Design review of the part shown in the three views and the two pictorial views. Dimensions are in mm from the part's minimum x, y and z. A direction names the side the tool comes from. Round coordinates to 2 decimals unless told otherwise and drop trailing zeros. Loops run counter-clockwise (first coordinate to the right, second up) from the corner with the lowest first, then second, coordinate; pieces in that order, holes last. Notation, with made-up numbers: M -6.75,54.5 L 52.25,54.5 A18 cw 52.25,68.5 Z; hole C 12,-22.5 d8. An arc over 180 degrees is marked long. One line per question, with ' | ' between items. Start each with the question number.
1) For the marked faces 5, 6, 7 and 8, list the 3-axis set-ups (+Z, -Z, +X, -X, +Y, -Y) from which the entire face can be reached by the end or side of a thin tool; tool diameter is ignored.
2) Mouldability with a two-part tool opening along X and no side actions: class the marked faces 1, 2, 3 and 4 as pulls with the +X half, pulls with the -X half, needs draft (parallel to the pull), parting line crosses it, or undercut.
3) We need section C-C (x = 29). Give the boundary of the cut face in (y, z).
4) For probe 1 along X at (y, z) = (1.25, 7.5); probe 2 along X at (y, z) = (4, 1); probe 3 along X at (y, z) = (3, 2.5), list the stretches that pass through material, from the lowest coordinate up. Write a range as from..to.
5) For pin 1 Ø4.5 at (x, z) = (28, 3) entering from +Y (1 decimal); pin 2 Ø2.5 at (x, z) = (5, 14) entering from +Y, all flat-tipped, find the tip position at first contact; note any pin that passes through.
6) We need section A-A (x = 7). Give the boundary of the cut face in (y, z).
7) We need section D-D (z = 1). Give the boundary of the cut face in (x, y).
8) We need section B-B (z = 11.5). Give the boundary of the cut face in (x, y), and give its area (3 significant figures).
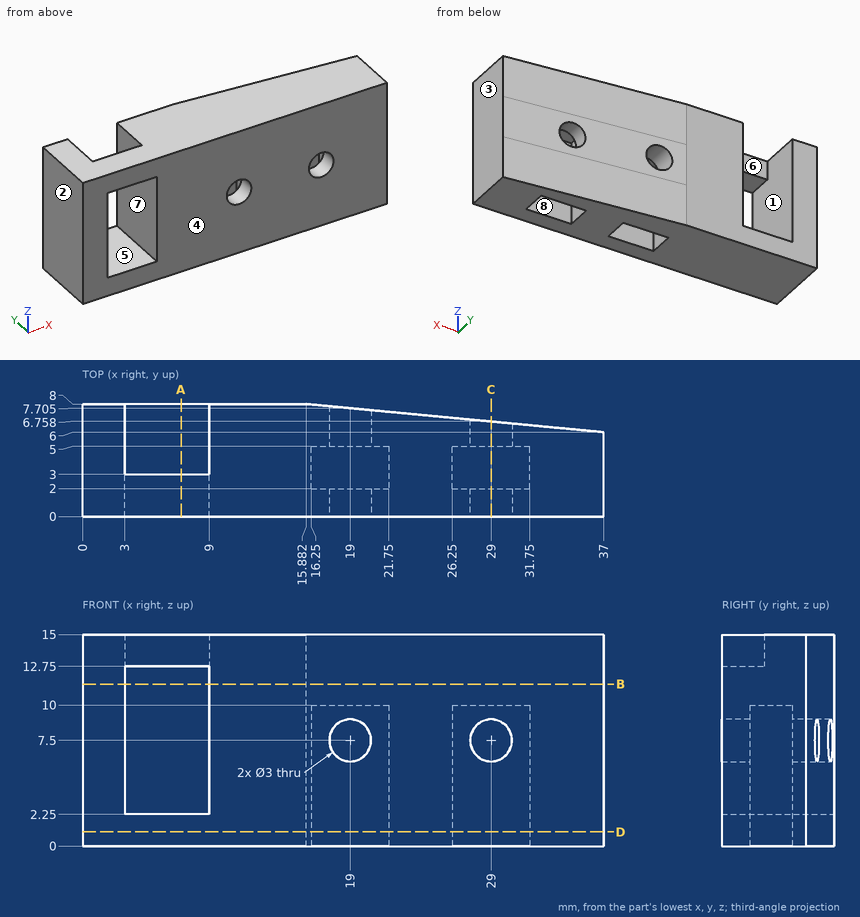
Answers below:
1) face 5: +Y, -Y | face 6: +Z, +Y | face 7: +Y | face 8: -Z
2) face 1: undercut | face 2: pulls with the -X half | face 3: pulls with the +X half | face 4: needs draft
3) outline: M 0,0 L 2,0 L 2,6 L 0,6 Z; M 0,9 L 2,9 L 2,10 L 5,10 L 5,9 L 6.76,9 L 6.76,15 L 0,15 Z; M 5,0 L 6.76,0 L 6.76,6 L 5,6 Z
4) probe 1: 0..3, 9..17.5, 20.5..27.5, 30.5..37 | probe 2: 0..16.25, 21.75..26.25, 31.75..37 | probe 3: 0..3, 9..16.25, 21.75..26.25, 31.75..37
5) pin 1: y = 7.1 | pin 2: y = 3
6) outline: M 0,0 L 8,0 L 8,2.25 L 0,2.25 Z; M 0,12.75 L 3,12.75 L 3,15 L 0,15 Z
7) outline: M 0,0 L 37,0 L 37,6 L 15.88,8 L 0,8 Z; hole M 16.25,2 L 21.75,2 L 21.75,5 L 16.25,5 Z; hole M 26.25,2 L 31.75,2 L 31.75,5 L 26.25,5 Z
8) outline: M 0,0 L 3,0 L 3,8 L 0,8 Z; M 9,0 L 37,0 L 37,6 L 15.88,8 L 9,8 Z | area: 227 mm^2
